Work out the finished part from the listing and answer in its coordinate system (mm). Round coordinates to 2 decimals unless told otherwise and drop trailing zeros. Write each loop counter-clockwise with the first axis right and the second up, starting at its lowest first coordinate (ties: lowest second). Pieces come first, ordered by that corner, then holes. Notation, with made-up numbers: M 35,87 L 46,87 A11 cw 46,93 Z; hole C 1,27 d10. An arc over 180 degrees is marked long. One line per item, written item: value. Start each with the question number.
Q1. Find section A-A (x = 85). Write down the section's boundary in (y, z).
Q2. Find section C-C (y = 2.75). Write down the section's boundary in (x, z), and give its area (3 significant figures).
Q3. Given pin 1 Ø6 at (x, z) = (-85, -45) entering from +Y, flat-ended and moving along its own axis, determine where the tip first touches the part or whether it passes through.
Q4. Find section B-B (z = -45). Write down the section's boundary in (x, y), and give its area (3 significant figures).
Q5. Consider probe 1 along X at (y, z) = (1.5, 45); probe 2 along Z at (x, y) = (85, 4.25); probe 3 along Z at (x, y) = (86, 3.25). Determine where each line is inside the solid, lowest interval first.
from build123d import *

# Parameters (mm, degrees)
ESQUISSE1_W                     = 200
ESQUISSE1_H                     = 120
BOSS_EXTRU_1_DEPTH              = 6.35
DIAM_TRE_DU_PER_AGE_10_0_10_1_D = 10
CONG_1_R                        = 10


with BuildPart() as part:
    # Esquisse1 → Boss.-Extru.1 (new body)
    with BuildSketch(Plane(origin=(0, 0, 0), x_dir=(1, 0, 0), z_dir=(0, 1, 0))):
        Rectangle(ESQUISSE1_W, ESQUISSE1_H)
    extrude(amount=BOSS_EXTRU_1_DEPTH)

    # Diamètre du perçage Ø10.0 (10)1 (through all)
    with Locations(Plane(origin=(0, 6.35, 0), x_dir=(1, 0, 0), z_dir=(0, 1, 0))):
        with Locations((-85, 45), (-85, -45), (85, -45), (85, 45)):
            Hole(DIAM_TRE_DU_PER_AGE_10_0_10_1_D / 2)

    # Congé1
    cong_1_edges = [part.edges().sort_by_distance(p)[0] for p in [
        (100, 3.175, 60),
        (-100, 3.175, 60),
        (-100, 3.175, -60),
        (100, 3.175, -60),
    ]]
    fillet(cong_1_edges, radius=CONG_1_R)


solid = part.part
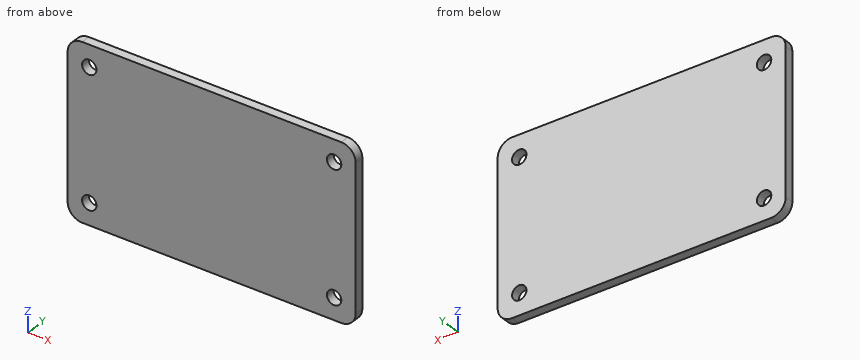
The answers:
1. outline: M 0,-60 L 6.35,-60 L 6.35,-50 L 0,-50 Z; M 0,-40 L 6.35,-40 L 6.35,40 L 0,40 Z; M 0,50 L 6.35,50 L 6.35,60 L 0,60 Z
2. outline: M -100,-50 A10 ccw -90,-60 L 90,-60 A10 ccw 100,-50 L 100,50 A10 ccw 90,60 L -90,60 A10 ccw -100,50 Z; hole C -85,-45 d10; hole C -85,45 d10; hole C 85,-45 d10; hole C 85,45 d10
2. area: 23,600 mm2
3. pin 1: through
4. outline: M -100,0 L -90,0 L -90,6.35 L -100,6.35 Z; M -80,0 L 80,0 L 80,6.35 L -80,6.35 Z; M 90,0 L 100,0 L 100,6.35 L 90,6.35 Z
4. area: 1,140 mm2
5. probe 1: -100 to -90, -80 to 80, 90 to 100
5. probe 2: -60 to -50, -40 to 40, 50 to 60
5. probe 3: -60 to -49.9, -40.1 to 40.1, 49.9 to 60
